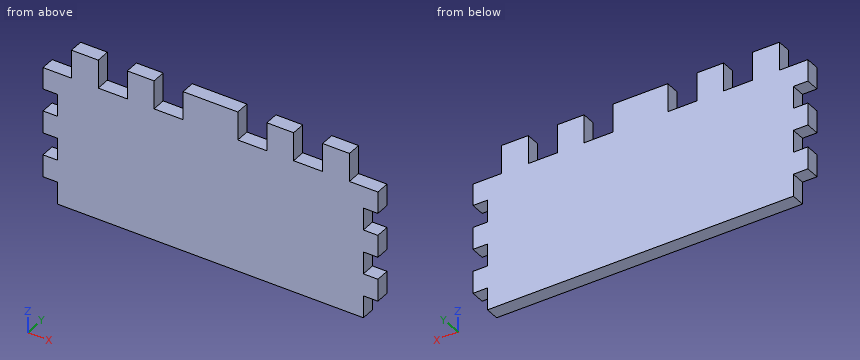
```python
from build123d import *

# Parameters (mm, degrees)
SKETCH1_W           = 76.2
SKETCH1_H           = 30.48
BOSS_EXTRUDE1_DEPTH = 3.175
SKETCH5_W           = 3.302
SKETCH5_H           = 5.08
CUT_EXTRUDE2_DEPTH  = 42.157602275
SKETCH6_W           = 76.2
SKETCH6_H           = 6.35
BOSS_EXTRUDE3_DEPTH = 3.175
SKETCH7_W           = 6.604
SKETCH7_H           = 6.604
CUT_EXTRUDE3_DEPTH  = 44.906932539


with BuildPart() as part:
    # Sketch1 → Boss-Extrude1 (new body)
    with BuildSketch(Plane(origin=(0, 0, 0), x_dir=(1, 0, 0), z_dir=(0, 1, 0))):
        Rectangle(SKETCH1_W, SKETCH1_H)
    extrude(amount=BOSS_EXTRUDE1_DEPTH)

    # Sketch5 → Cut-Extrude2 (cut, through all)
    with BuildSketch(Plane(origin=(0, 3.175, 0), x_dir=(1, 0, 0), z_dir=(0, 1, 0))):
        with Locations((-36.449, 2.54)):
            Rectangle(SKETCH5_W, SKETCH5_H)
        with Locations((-36.449, 12.7)):
            Rectangle(SKETCH5_W, SKETCH5_H)
        with Locations((-36.449, -7.62)):
            Rectangle(SKETCH5_W, SKETCH5_H)
        with Locations((36.449, -7.62)):
            Rectangle(SKETCH5_W, SKETCH5_H)
        with Locations((36.449, 2.54)):
            Rectangle(SKETCH5_W, SKETCH5_H)
        with Locations((36.449, 12.7)):
            Rectangle(SKETCH5_W, SKETCH5_H)
    extrude(amount=-CUT_EXTRUDE2_DEPTH, mode=Mode.SUBTRACT)

    # Sketch6 → Boss-Extrude3 (add)
    with BuildSketch(Plane(origin=(0, 3.175, 0), x_dir=(1, 0, 0), z_dir=(0, 1, 0))):
        with Locations((0, -18.415)):
            Rectangle(SKETCH6_W, SKETCH6_H)
    extrude(amount=-BOSS_EXTRUDE3_DEPTH)

    # Sketch7 → Cut-Extrude3 (cut, through all)
    with BuildSketch(Plane(origin=(0, 3.175, 0), x_dir=(1, 0, 0), z_dir=(0, 1, 0))):
        with Locations((-34.925, -18.415)):
            Rectangle(SKETCH7_W, SKETCH7_H)
        with Locations((-22.225, -18.415)):
            Rectangle(SKETCH7_W, SKETCH7_H)
        with Locations((-9.525, -18.415)):
            Rectangle(SKETCH7_W, SKETCH7_H)
        with Locations((9.525, -18.415)):
            Rectangle(SKETCH7_W, SKETCH7_H)
        with Locations((22.225, -18.415)):
            Rectangle(SKETCH7_W, SKETCH7_H)
        with Locations((34.925, -18.415)):
            Rectangle(SKETCH7_W, SKETCH7_H)
    extrude(amount=-CUT_EXTRUDE3_DEPTH, mode=Mode.SUBTRACT)


solid = part.part
```
Build history of the part. All positions in model axes, mm. Give positions to 0.01 mm unless a question says otherwise; leave off trailing zeros. Order: outer loops, then holes, each group sorted by start corner. A loop starts at its lowest first (then second) coordinate and runs counter-clockwise, first axis right, second up. Notation, with made-up numbers: M 70.5,33.25 L 85.5,33.25 A27 cw 85.5,62.25 Z; hole C 52,81 d5. An arc over 180 degrees is marked long. Write item = value, one per line. Start each with the question number.
(1) Slice it at A-A on z = 9. Write the cut outline in (x, y) (3 decimals), plus the area to 3 significant figures.
(2) Pin check, flat tips, straight feed: pin 1 Ø1 at (y, z) = (2, 19.5) entering from -X; pin 2 Ø1 at (x, y) = (35.5, 1) entering from +Z; pin 3 Ø1.6 at (x, y) = (36, 1.5) entering from -Z. Stop position of each tip, or through.
(3) Probe L1, parallel to X at y = 0.65, z = 15.5; L2, parallel to X at y = 0.7, z = -14; L3, parallel to Z at x = -7.5, y = 2.8. List the from-to ranges inside material, lowest first. Write a range as [from, to].
(4) Slice it at B-B on x = -10. Write the cut outline in (y, z) (3 decimals).
Responses:
q1.outline = M -34.798,0 L 34.798,0 L 34.798,3.175 L -34.798,3.175 Z
q1.area = 221 mm2
q2.pin_1 = -31.62
q2.pin_2 = 15.11
q2.pin_3 = -10.16
q3.L1 = [-31.62, -25.53], [-18.92, -12.83], [-6.22, 6.22], [12.83, 18.92], [25.53, 31.62]
q3.L2 = [-34.8, 34.8]
q3.L3 = [-15.24, 15.11]
q4.outline = M 0,-15.24 L 3.175,-15.24 L 3.175,15.113 L 0,15.113 Z
